from build123d import *

# Parameters (mm, degrees)
PAD004_DEPTH            = 6
THICKNESS_T             = -0.2
SKETCH016_W             = 0.1
SKETCH016_H             = 1
PAD005_DEPTH            = 1
SKETCH017_W             = 0.5
SKETCH017_H             = 0.5
PAD006_DEPTH            = 0.4
SKETCH018_W             = 0.32
SKETCH018_H             = 1.35
PAD007_DEPTH            = 0.1
BODY002_ROLL_ANGLE      = 90
BODY002_PLACEMENT_ANGLE = 90


with BuildPart() as part:
    # Sketch015 → Pad004 (new body)
    with BuildSketch(Plane.XY):
        Polygon((0, 0), (6.5, 0), (7, -1), (6, -2.6), (0.5, -2.6), (-0.5, -1), align=None)
    extrude(amount=PAD004_DEPTH)

    # Thickness
    thickness_openings = [part.faces().sort_by_distance(p)[0] for p in [
        (3.25, -1.25728, 6),
    ]]
    offset(amount=THICKNESS_T, openings=thickness_openings)

    # Sketch016 (on Face5 of Thickness) → Pad005 (join)
    with BuildSketch(Plane.XZ.offset(2.6)):
        with Locations((5.95, 3)):
            Rectangle(SKETCH016_W, SKETCH016_H)
        with Locations((0.55, 3)):
            Rectangle(SKETCH016_W, SKETCH016_H)
    extrude(amount=PAD005_DEPTH)

    # Sketch017 (on Face7 of Pad005) → Pad006 (join)
    with BuildSketch(Plane.XZ.offset(2.6)):
        with Locations((1.35, 0.25)):
            Rectangle(SKETCH017_W, SKETCH017_H)
        with Locations((5.15, 0.25)):
            Rectangle(SKETCH017_W, SKETCH017_H)
    extrude(amount=PAD006_DEPTH)

    # Sketch018 (on Face7 of Pad006) → Pad007 (join)
    with BuildSketch(Plane.XZ.offset(2.6)):
        with Locations((1.81, -0.025)):
            Rectangle(SKETCH018_W, SKETCH018_H)
        with Locations((2.53, -0.025)):
            Rectangle(SKETCH018_W, SKETCH018_H)
        with Locations((3.25, -0.025)):
            Rectangle(SKETCH018_W, SKETCH018_H)
        with Locations((3.97, -0.025)):
            Rectangle(SKETCH018_W, SKETCH018_H)
        with Locations((4.69, -0.025)):
            Rectangle(SKETCH018_W, SKETCH018_H)
    extrude(amount=PAD007_DEPTH)


with BuildPart() as part_1:
    # Body002 roll: moved
    add(part.part.rotate(Axis((0, 0, 0), (1, 0, 0)), BODY002_ROLL_ANGLE))


with BuildPart() as part_2:
    # Body002 placement: moved
    add(part_1.part.moved(Location((86, -3, 12))).rotate(Axis((86, -3, 12), (0, 0, 1)), BODY002_PLACEMENT_ANGLE))


solid = part_2.part
The model under review builds one solid part; all positions refer to its coordinate system, in mm. A direction names the side the tool comes from. Round coordinates to 2 decimals unless told otherwise and drop trailing zeros. Write each loop counter-clockwise with the first axis right and the second up, starting at its lowest first coordinate (ties: lowest second). Pieces come first, ordered by that corner, then holes. Notation, with made-up numbers: (-21.75, 83.25) -> (-5.75, 83.25) arc R29 cw to (-5.75, 118.25) -> close; hole circle Ø7 at (-21.5, 43.25). An arc over 180 degrees is marked (long way). Answer as a JSON object with one key per item and string values.
1. Clearance check with flat-ended pins moving along their axes: pin 1 (1.1 mm diameter, centred on x = 89, z = 9, fed in from -Y); pin 2 (1.1 mm diameter, centred on x = 89, z = 8.5, fed in from +Y). State where each tip first meets the part, or that it passes through.
Results found:
{"pin 1": "stops at y = -2.59", "pin 2": "stops at y = 3"}
2. Machinability: for faces 4 (the face through (88.958, -3.254, 11.493)), 5 (the face through (86.2, 0, 11)), which of the approach directions +Z, -Z, +X, -X, +Y, -Y give a long, thin tool a straight path to every point of the face, cutting with its end or side? Answer none if there is none.
Results found:
{"face 4": "+Z, +X, -X, -Y", "face 5": "+X"}
3. We need section D-D on x = 89. State the section outline as (y, z) points.
Results found:
{"outline": "(-3.5, 11) -> (-2.5, 9.4) -> (-2.5, 8.4) -> (-2.4, 8.4) -> (-2.4, 9.4) -> (2.9, 9.4) -> (2.9, 8.4) -> (3, 8.4) -> (3, 9.4) -> (4, 11) -> (3.5, 12) -> (-3, 12) -> close; hole (-3.27, 11.01) -> (-2.39, 9.6) -> (2.89, 9.6) -> (3.77, 11.01) -> (3.38, 11.8) -> (-2.88, 11.8) -> close"}
4. The part is to be moulded in two halves that separate along Z. For faces 1 (the face through (89.059, -2.824, 10.296)), 2 (the face through (89, 0, 12)), 3 (the face through (89, 3.5, 10.2)), say which applies: pulls with the +Z half, pulls with the -Z half, needs draft (parallel to the pull), parting line crosses it, or undercut.
Results found:
{"face 1": "undercut", "face 2": "pulls with the +Z half", "face 3": "pulls with the -Z half"}
5. To check wall thickness, follow line 1 along Z through (x, y) = (91, 2.5); line 2 along Y through (x, z) = (88, 10.6); line 3 along X through (y, z) = (-1, 10.25). State the ranges of each line that lie inside material, in increasing order.
Results found:
{"line 1": "z = 9.4 to 9.6, 11.8 to 12", "line 2": "y = -3.25 to -3.01, 3.51 to 3.75", "line 3": "x = 86 to 86.2"}
6. We need section B-B on y = -1.5. State the section outline as (x, z) points.
Results found:
{"outline": "(86, 9) -> (86.5, 9) -> (86.5, 9.4) -> (92, 9.4) -> (92, 9.6) -> (86.2, 9.6) -> (86.2, 11.8) -> (92, 11.8) -> (92, 12) -> (86, 12) -> close"}
7. We need section A-A on x = 87. State the section outline as (y, z) points, and give its area (3 significant figures).
Results found:
{"outline": "(-3.5, 11) -> (-2.5, 9.4) -> (3, 9.4) -> (4, 11) -> (3.5, 12) -> (-3, 12) -> close; hole (-3.27, 11.01) -> (-2.39, 9.6) -> (2.89, 9.6) -> (3.77, 11.01) -> (3.38, 11.8) -> (-2.88, 11.8) -> close", "area": "3.46 mm^2"}
8. We need section C-C on z = 11.25. State the section outline as (x, y) points (3 decimals).
Results found:
{"outline": "(86, -3.375) -> (92, -3.375) -> (92, -3.151) -> (86.2, -3.151) -> (86.2, 3.651) -> (92, 3.651) -> (92, 3.875) -> (86, 3.875) -> close"}
